```python
from build123d import *

# Parameters (mm, degrees)
F0_W      = 269.875
F0_H      = 273.05
F1_DEPTH  = 19.05
F3_DEPTH  = 12.7
F5_DEPTH  = 19.05
F6_W      = 3.175
F6_H      = 273.05
F7_DEPTH  = 19.05
F8_W      = 263.525
F8_H      = 3.175
F9_DEPTH  = 19.05
F11_DEPTH = 6.35
F13_DEPTH = 6.35
F14_W     = 263.525
F14_H     = 3.175
F15_DEPTH = 19.05


# Not quite as in the source:
# - ends of sketch curves that miss each other by under 0.0002 mm in the source are joined


with BuildPart() as f1:
    # F0 (on Top) → F1 (new body)
    with BuildSketch(Plane.XY):
        Rectangle(F0_W, F0_H)
    extrude(amount=F1_DEPTH)

    # F2 (on face) → F3 (cut)
    with BuildSketch(Plane.XY.offset(19.05)):
        with BuildLine():
            ThreePointArc((55.5625, 107.0944960946), (84.6752951993, 85.9448479137), (106.2558233698, 57.15))
            Line((106.2558233698, 57.15), (125.4125, 57.15))
            Line((125.4125, 57.15), (125.4125, 127))
            Line((125.4125, 127), (55.5625, 127))
            Line((55.5625, 127), (55.5625, 107.0944960946))
        make_face()
        with BuildLine():
            Line((-125.4125, 57.15), (-106.2558233698, 57.15))
            ThreePointArc((-106.2558233698, 57.15), (-84.6752951993, 85.9448479137), (-55.5625, 107.0944960946))
            Line((-55.5625, 107.0944960946), (-55.5625, 127))
            Line((-55.5625, 127), (-125.4125, 127))
            Line((-125.4125, 127), (-125.4125, 57.15))
        make_face()
    extrude(amount=-F3_DEPTH, mode=Mode.SUBTRACT)

    # F4 (on face) → F5 (cut, through all)
    with BuildSketch(Plane.XY.offset(19.05)):
        with BuildLine():
            Line((-106.3625, -107.9627), (-106.3625, -71.4977328139))
            ThreePointArc((-106.3625, -71.4977328139), (-115.8875, -61.468), (-125.4125, -71.4977328139))
            Line((-125.4125, -71.4977328139), (-125.4125, -107.9627))
            Line((-125.4125, -107.9627), (-125.3998, -107.9627))
            ThreePointArc((-125.3998, -107.9627), (-115.8875, -117.475), (-106.3752, -107.9627))
            Line((-106.3752, -107.9627), (-106.3625, -107.9627))
        make_face()
        with BuildLine():
            ThreePointArc((125.4125, -71.4977328139), (115.8875, -61.468), (106.3625, -71.4977328139))
            Line((106.3625, -71.4977328139), (106.3625, -107.228528768))
            ThreePointArc((106.3625, -107.228528768), (115.8875, -117.475), (125.4125, -107.228528768))
            Line((125.4125, -107.228528768), (125.4125, -71.4977328139))
        make_face()
    extrude(amount=-F5_DEPTH, mode=Mode.SUBTRACT)

    # F6 (on face) → F7 (cut, through all)
    with BuildSketch(Plane.XY.offset(19.05)):
        with Locations((-133.35, 0)):
            Rectangle(F6_W, F6_H)
        with Locations((133.35, 0)):
            Rectangle(F6_W, F6_H)
    extrude(amount=-F7_DEPTH, mode=Mode.SUBTRACT)

    # F8 (on face) → F9 (cut, through all)
    with BuildSketch(Plane.XY.offset(19.05)):
        with Locations((0, 134.9375)):
            Rectangle(F8_W, F8_H)
    extrude(amount=-F9_DEPTH, mode=Mode.SUBTRACT)

    # F10 (on face) → F11 (cut)
    with BuildSketch(Plane.XY.offset(19.05)):
        with BuildLine():
            Line((24.2490875216, -2.6255133905), (24.253090398, -0.6476470458))
            ThreePointArc((24.253090398, -0.6476470458), (-1.7785482929, 22.6185422911), (-24.13, -4.2026132727))
            Line((-24.13, -4.2026132727), (-24.13, -61.468))
            Line((-24.13, -61.468), (-115.8875, -61.468))
            ThreePointArc((-115.8875, -61.468), (-108.9715552829, -64.4377908989), (-106.3625, -71.4977328139))
            Line((-106.3625, -71.4977328139), (-106.3625, -107.9627))
            Line((-106.3625, -107.9627), (-106.3752, -107.9627))
            ThreePointArc((-106.3752, -107.9627), (-109.1568025344, -114.6844232103), (-115.8748084893, -117.4749915334))
            Line((-115.8748084893, -117.4749915334), (115.8875, -117.475))
            ThreePointArc((115.8875, -117.475), (108.892576882, -114.4269988445), (106.3625, -107.228528768))
            Line((106.3625, -107.228528768), (106.3625, -71.4977328139))
            ThreePointArc((106.3625, -71.4977328139), (108.9715552829, -64.4377908989), (115.8875, -61.468))
            Line((115.8875, -61.468), (24.13, -61.468))
            Line((24.13, -61.468), (24.2490875216, -2.6255133905))
        make_face()
    extrude(amount=-F11_DEPTH, mode=Mode.SUBTRACT)

    # F12 (on face) → F13 (cut)
    with BuildSketch(Plane.XY.offset(19.05)):
        with BuildLine():
            Line((119.0726616849, 57.15), (112.5956616849, 57.15))
            Line((112.5956616849, 57.15), (112.5956616849, -61.468))
            Line((112.5956616849, -61.468), (115.8875, -61.468))
            ThreePointArc((115.8875, -61.468), (117.5034429216, -61.6058888442), (119.0726616849, -62.0155683919))
            Line((119.0726616849, -62.0155683919), (119.0726616849, 57.15))
        make_face()
        with BuildLine():
            Line((-115.8341616849, -61.468), (-112.5956616849, -61.468))
            Line((-112.5956616849, -61.468), (-112.5956616849, 57.15))
            Line((-112.5956616849, 57.15), (-119.0726616849, 57.15))
            Line((-119.0726616849, 57.15), (-119.0726616849, -61.468))
            Line((-119.0726616849, -61.468), (-119.0726616849, -62.0155683919))
            ThreePointArc((-119.0726616849, -62.0155683919), (-117.4763944176, -61.6058567373), (-115.8341616849, -61.468))
        make_face()
    extrude(amount=-F13_DEPTH, mode=Mode.SUBTRACT)

    # F14 (on face) → F15 (cut, through all)
    with BuildSketch(Plane.XY.offset(19.05)):
        with Locations((0, -134.9375)):
            Rectangle(F14_W, F14_H)
    extrude(amount=-F15_DEPTH, mode=Mode.SUBTRACT)


solid = f1.part
```
Here's how the part is built. I have some questions about the finished solid (model axes, mm). A direction names the side the tool comes from. Give positions to 0.01 mm unless a question says otherwise; leave off trailing zeros. Loops run counter-clockwise (first coordinate to the right, second up) from the corner with the lowest first, then second, coordinate; pieces in that order, holes last. Notation, with made-up numbers: M 58.5,-3 L 67.5,-3 A18 ccw 67.5,32 Z; hole C 83,58.5 d8. An arc over 180 degrees is marked long. Return JSON: item names as keys, results as strings.
Item 1: I'm going to push a flat-ended pin straight in: pin 1 Ø12 at (x, y) = (-7.5, 97) entering from -Z. Where does the tip first touch, or does it pass through?
A:
{"pin 1": "stops at z = 0"}
Item 2: Imagine slicing it at A-A on x = 0. List the corners of the cut face in (y, z) for me (3 decimals), then the cut area to 3 significant figures.
A:
{"outline": "M -133.35,0 L 133.35,0 L 133.35,19.05 L 22.684,19.05 L 22.684,12.7 L -117.475,12.7 L -117.475,19.05 L -133.35,19.05 Z", "area": "4,190 mm^2"}
Item 3: On a 3-axis mill with a long thin cutter (end or side, diameter ignored), from which of +Z, -Z, +X, -X, +Y, -Y can I reach the whole of each face in a straight line? I mean faces 4 (the cylindrical face through (119.45, -62.16, 7.54)), 5 (the flat face through (69, -61.468, 16)). Say none if no direction works.
A:
{"face 4": "+Z, -Z", "face 5": "+Z"}
Item 4: Imagine slicing it at B-B on y = 83. List the corners of the cut face in (x, z) for me.
A:
{"outline": "M -131.76,0 L 131.76,0 L 131.76,19.05 L 125.41,19.05 L 125.41,6.35 L 87.56,6.35 L 87.56,19.05 L -87.56,19.05 L -87.56,6.35 L -125.41,6.35 L -125.41,19.05 L -131.76,19.05 Z"}
Item 5: Imagine slicing it at C-C on x = -67. List the corners of the cut face in (y, z) for me (3 decimals), then the cut area to 3 significant figures.
A:
{"outline": "M -133.35,0 L 133.35,0 L 133.35,19.05 L 127,19.05 L 127,6.35 L 100.337,6.35 L 100.337,19.05 L -61.468,19.05 L -61.468,12.7 L -117.475,12.7 L -117.475,19.05 L -133.35,19.05 Z", "area": "4,390 mm^2"}
Item 6: Please list where these lines run through material, in increasing order: line 1 (X direction, y = -25, z = 16); line 2 (X direction, y = -88, z = 10.25); line 3 (Y direction, x = -93.5, z = 12.75) (3 decimals).
A:
{"line 1": "x = -131.76 to -119.07, -112.6 to -24.13, 24.2 to 112.6, 119.07 to 131.76", "line 2": "x = -131.76 to -125.41, -106.36 to 106.36, 125.41 to 131.76", "line 3": "y = -133.35 to -117.475, -61.468 to 76.251, 127 to 133.35"}
Item 7: Thinking about a two-plate mould opening in X: for faces 1 (the flat face through (-131.762, -2, 10)), 2 (the cylindrical face through (84.314, 86.299, 12.789)), 3 (the flat face through (98, 100, 6.35)), which applies, released by +X, released by -X, zero draft, split by the parting line, or undercut?
A:
{"face 1": "released by -X", "face 2": "undercut", "face 3": "undercut"}
Item 8: Imagine slicing it at D-D on y = 9. List the corners of the cut face in (x, z) for me, then the cut area to 3 significant figures.
A:
{"outline": "M -131.76,0 L 131.76,0 L 131.76,19.05 L 119.07,19.05 L 119.07,12.7 L 112.6,12.7 L 112.6,19.05 L 21.84,19.05 L 21.84,12.7 L -21.84,12.7 L -21.84,19.05 L -112.6,19.05 L -112.6,12.7 L -119.07,12.7 L -119.07,19.05 L -131.76,19.05 Z", "area": "4,660 mm^2"}
